Check sheet for the modelled part. Datum: model origin and axes. Units: mm. Face numbers are marked on the shaded views. Round coordinates to 2 decimals unless told otherwise and drop trailing zeros. Write each loop counter-clockwise with the first axis right and the second up, starting at its lowest first coordinate (ties: lowest second). Pieces come first, ordered by that corner, then holes.
Item 1: Cross-section at C-C on z = -7.5. Enter the section's corners in (x, y), plus the area to 3 significant figures.
Item 2: Release check for a two-part mould opening along Y. For the marked faces 1 and 2 record: +Y half, -Y half, draft (parallel to the pull), parting line (faces both ways), or undercut.
Item 3: Cross-section at A-A on x = 10.5. Enter the section's corners in (y, z) (3 decimals).
Item 4: Cross-section at B-B on y = 23. Enter the section's corners in (x, z).
Item 5: Go/stop test with flat-tipped pins: pin 1 Ø10 at (x, y) = (18.5, -13.5) entering from -Z; pin 2 Ø5 at (x, z) = (20.5, 1.5) entering from +Y (3 decimals); pin 3 Ø6 at (x, z) = (14.5, -4) entering from -Y. Record where each tip stops, or that it passes through.
Item 6: Cross-section at D-D on x = 1.5. Enter the section's corners in (y, z) (3 decimals), plus the area to 3 significant figures.
Item 7: Material ranges on line 1 (Y direction, x = 7.5, z = 0) (3 decimals); line 2 (Z direction, x = 13.75, y = 0.5); line 3 (Y direction, x = 11.25, z = 0) (3 decimals), recorded low to high.
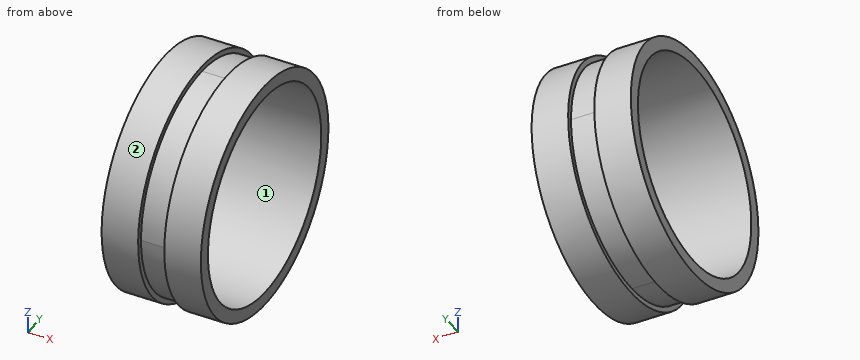
from build123d import *

# Parameters (mm, degrees)
SKETCH1_R           = 28.575
SKETCH1_R_2         = 25.4
BOSS_EXTRUDE1_DEPTH = 24.13


with BuildPart() as part:
    # Sketch1 → Boss-Extrude1 (new body)
    with BuildSketch(Plane(origin=(0, 0, 0), x_dir=(0, 0, -1), z_dir=(1, 0, 0))):
        with Locations(Location((0, 0, 0), (0, 0, 180))):
            Circle(SKETCH1_R)
        with Locations(Location((0, 0, 0), (0, 0, 180))):
            Circle(SKETCH1_R_2, mode=Mode.SUBTRACT)
    extrude(amount=BOSS_EXTRUDE1_DEPTH)

    # Cut-Sweep1: sweep along a curve in space
    with BuildLine() as cut_sweep1_path:
        ThreePointArc((24.13, 0, -28.575), (24.13, 20.205576272, -20.205576272), (24.13, 28.575, 0))
        ThreePointArc((24.13, 28.575, 0), (24.13, 20.205576272, 20.205576272), (24.13, 0, 28.575))
        ThreePointArc((24.13, 0, 28.575), (24.13, -20.205576272, 20.205576272), (24.13, -28.575, 0))
        ThreePointArc((24.13, -28.575, 0), (24.13, -20.205576272, -20.205576272), (24.13, 0, -28.575))
    # Sketch2 → Cut-Sweep1 (sweep, cut)
    with BuildSketch(Plane.XY):
        Polygon((15.24, 28.575), (15.24, 27.305), (8.89, 27.305), (8.89, 28.575), (8.89, 30.628551977), (15.24, 30.628551977), align=None)
    sweep(path=cut_sweep1_path.line, mode=Mode.SUBTRACT)


solid = part.part
Response values:
1. outline: (0, -27.57) - (8.89, -27.57) - (8.89, -26.25) - (15.24, -26.25) - (15.24, -27.57) - (24.13, -27.57) - (24.13, -24.27) - (0, -24.27) - close; (0, 24.27) - (24.13, 24.27) - (24.13, 27.57) - (15.24, 27.57) - (15.24, 26.25) - (8.89, 26.25) - (8.89, 27.57) - (0, 27.57) - close
1. area: 143 mm2
2. face 1: undercut
2. face 2: parting line
3. outline: circle Ø54.61 at (0, 0); hole circle Ø50.8 at (0, 0)
4. outline: (0, -16.96) - (8.89, -16.96) - (8.89, -14.72) - (15.24, -14.72) - (15.24, -16.96) - (24.13, -16.96) - (24.13, -10.78) - (0, -10.78) - close; (0, 10.78) - (24.13, 10.78) - (24.13, 16.96) - (15.24, 16.96) - (15.24, 14.72) - (8.89, 14.72) - (8.89, 16.96) - (0, 16.96) - close
5. pin 1: stops at z = -27.28
5. pin 2: stops at y = 28.575
5. pin 3: stops at y = -28.55
6. outline: circle Ø57.15 at (0, 0); hole circle Ø50.8 at (0, 0)
6. area: 538 mm2
7. line 1: y = -28.575 to -25.4, 25.4 to 28.575
7. line 2: z = -27.3 to -25.4, 25.4 to 27.3
7. line 3: y = -27.305 to -25.4, 25.4 to 27.305
